Verification items for the finished model (mm, model axes). Coordinates: 2 decimals unless noted, no trailing zeros. Write each loop counter-clockwise with the first axis right and the second up, starting at its lowest first coordinate (ties: lowest second). Pieces come first, ordered by that corner, then holes. Notation, with made-up numbers: M 59,8 L 75,8 A8 ccw 75,20 Z; hole C -3,81.25 d9. An arc over 180 degrees is marked long. One line per item, written item: value.
Autodesk Inventor part; units mm, degrees
ref_plane "YZ Plane" through (0, 0, 0) normal (1, 0, 0) x (0, 1, 0)
ref_plane "XZ Plane" through (0, 0, 0) normal (0, 1, 0) x (-1, 0, 0)
ref_plane "XY Plane" through (0, 0, 0) normal (0, 0, 1) x (1, 0, 0)
sketch "Sketch1" plane through (0, 0, 0) normal (0, 0, 1) x (1, 0, 0)
  line L0 (0, 0) -> (0, 203.2)
  line L1 (0, 203.2) -> (50.8, 203.2)
  line L2 (50.8, 203.2) -> (50.8, 0)
  line L3 (50.8, 0) -> (0, 0)
  dimension "d0" = 203.2
  dimension "d1" = 50.8
extrude "Extrusion1" add sketch "Sketch1" along normal blind 12.7
sketch "Sketch2" plane through (50.8, 0, 0) normal (1, 0, 0) x (0, 0, -1)
  circle A0 centre (-6.35, 185.7787) radius 3.175
  line L0 (0, 203.2) -> (0, 0)
  dimension "d4" = 6.35
  dimension "d7" = 6.35
extrude "Extrusion2" cut sketch "Sketch2" against normal blind 127
properties part number "Bar"
Item 1: Go/stop test with a flat-tipped pin: P1, Ø5, axis at y = 185.78, z = 6.35, coming from the -X side. Record where the tip stops, or that it passes through.
The answers:
P1: passes through
Item 2: Cross-section at A-A, the plane z = 6.35. Enter the section's corners in (x, y).
The answers:
outline: M 0,0 L 50.8,0 L 50.8,182.6 L 0,182.6 Z; M 0,188.95 L 50.8,188.95 L 50.8,203.2 L 0,203.2 Z
Item 3: Draft check along Z on faces 1 (the face through (26, 0, 6)), 2 (the face through (25.756, 188.927, 6.763)), 3 (the face through (25, 103, 12.7)). Enter one of: released by +Z, released by -Z, zero draft, split by the parting line, or undercut.
The answers:
face 1: zero draft
face 2: undercut
face 3: released by +Z
Item 4: Scan lines: line 1 (Y direction, x = 40, z = 6.35); line 2 (Y direction, x = 26, z = 4.5). Record each from-to range of solid material in increasing order.
The answers:
line 1: y = 0 to 182.6, 188.95 to 203.2
line 2: y = 0 to 183.2, 188.36 to 203.2
